from build123d import *

# Parameters (mm, degrees)
SKETCH_1_R      = 1.6
EXTRUDE_1_DEPTH = 3
CHAMFER_1_SIZE  = 4


with BuildPart() as part:
    # 草图1 → 凸台-拉伸1 (new body)
    with BuildSketch(Plane.XY):
        Polygon((-20.3, 16.9), (-35.3, 16.9), (-35.3, 8), (-31.3, 4), (-31.3, -6), (-35.3, -10), (-35.3, -18), (-31.3, -22), (-31.3, -32), (-35.3, -36), (-35.3, -52.9), (-20.3, -52.9), (-14.587407973, -56.9), (-8.874815946, -52.9), (11.874815946, -52.9), (17.587407973, -56.9), (23.3, -52.9), (23.3, -21), (20.3, -18), (23.3, -15), (23.3, 16.9), (17.587407973, 20.9), (11.874815946, 16.9), (-8.874815946, 16.9), (-14.587407973, 20.9), align=None)
        with Locations((-27.8, -47)):
            Circle(SKETCH_1_R, mode=Mode.SUBTRACT)
        with Locations((-27.8, -39)):
            Circle(SKETCH_1_R, mode=Mode.SUBTRACT)
        with BuildLine():
            ThreePointArc((-20.8, -30), (-23.3, -32.5), (-25.8, -30))
            Line((-25.8, -30), (-25.8, -24))
            ThreePointArc((-25.8, -24), (-23.3, -21.5), (-20.8, -24))
            Line((-20.8, -24), (-20.8, -30))
        make_face(mode=Mode.SUBTRACT)
        with BuildLine():
            Line((13.2, -46.9), (-13.2, -46.9))
            ThreePointArc((-13.2, -46.9), (-14.25, -47.95), (-15.3, -46.9))
            Line((-15.3, -46.9), (-15.3, -25.1))
            ThreePointArc((-15.3, -25.1), (-14.25, -24.05), (-13.2, -25.1))
            Line((-13.2, -25.1), (13.2, -25.1))
            ThreePointArc((13.2, -25.1), (14.25, -24.05), (15.3, -25.1))
            Line((15.3, -25.1), (15.3, -46.9))
            ThreePointArc((15.3, -46.9), (14.25, -47.95), (13.2, -46.9))
        make_face(mode=Mode.SUBTRACT)
        with Locations((-27.8, -14)):
            Circle(SKETCH_1_R, mode=Mode.SUBTRACT)
        with BuildLine():
            Line((-25.8, -4), (-25.8, 2))
            ThreePointArc((-25.8, 2), (-23.3, 4.5), (-20.8, 2))
            Line((-20.8, 2), (-20.8, -4))
            ThreePointArc((-20.8, -4), (-23.3, -6.5), (-25.8, -4))
        make_face(mode=Mode.SUBTRACT)
        with Locations((-27.8, 11)):
            Circle(SKETCH_1_R, mode=Mode.SUBTRACT)
        with BuildLine():
            Line((13.2, -10.9), (-13.2, -10.9))
            ThreePointArc((-13.2, -10.9), (-14.25, -11.95), (-15.3, -10.9))
            Line((-15.3, -10.9), (-15.3, 10.9))
            ThreePointArc((-15.3, 10.9), (-14.25, 11.95), (-13.2, 10.9))
            Line((-13.2, 10.9), (13.2, 10.9))
            ThreePointArc((13.2, 10.9), (14.25, 11.95), (15.3, 10.9))
            Line((15.3, 10.9), (15.3, -10.9))
            ThreePointArc((15.3, -10.9), (14.25, -11.95), (13.2, -10.9))
        make_face(mode=Mode.SUBTRACT)
    extrude(amount=EXTRUDE_1_DEPTH)

    # 倒角1
    chamfer_1_edges = [part.edges().sort_by_distance(p)[0] for p in [
        (-35.3, 16.9, 1.5),
        (-35.3, -52.9, 1.5),
    ]]
    chamfer(chamfer_1_edges, length=CHAMFER_1_SIZE)


solid = part.part
Build history of the part. All positions in model axes, mm. A direction names the side the tool comes from. Round coordinates to 2 decimals unless told otherwise and drop trailing zeros. Write each loop counter-clockwise with the first axis right and the second up, starting at its lowest first coordinate (ties: lowest second). Pieces come first, ordered by that corner, then holes. Notation, with made-up numbers: (79.5, 46.25) -> (120.5, 46.25) arc R15 cw to (120.5, 70.25) -> close; hole circle Ø3 at (55, 69). An arc over 180 degrees is marked (long way). Use one line per item in the form item = value.
Q1. Band-saw the part on B-B, the plane y = -39. Write the cut outline in (x, z).
Conclusion:
outline = (-35.3, 0) -> (-29.4, 0) -> (-29.4, 3) -> (-35.3, 3) -> close; (-26.2, 0) -> (-15.3, 0) -> (-15.3, 3) -> (-26.2, 3) -> close; (15.3, 0) -> (23.3, 0) -> (23.3, 3) -> (15.3, 3) -> close
Q2. Band-saw the part on D-D, the plane x = -27.8. Write the cut outline in (y, z).
Conclusion:
outline = (-52.9, 0) -> (-48.6, 0) -> (-48.6, 3) -> (-52.9, 3) -> close; (-45.4, 0) -> (-40.6, 0) -> (-40.6, 3) -> (-45.4, 3) -> close; (-37.4, 0) -> (-15.6, 0) -> (-15.6, 3) -> (-37.4, 3) -> close; (-12.4, 0) -> (9.4, 0) -> (9.4, 3) -> (-12.4, 3) -> close; (12.6, 0) -> (16.9, 0) -> (16.9, 3) -> (12.6, 3) -> close
Q3. Drill centre lines: L1, parallel to X at y = -0.5, z = 1.6; L2, parallel to Y at x = 0, z = 1.35; L3, parallel to Y at x = -27.8, z = 0.85. Where is each one in solid material? Low to high.
Conclusion:
L1 = -31.3 to -25.8, -20.8 to -15.3, 15.3 to 23.3
L2 = -52.9 to -46.9, -25.1 to -10.9, 10.9 to 16.9
L3 = -52.9 to -48.6, -45.4 to -40.6, -37.4 to -15.6, -12.4 to 9.4, 12.6 to 16.9
Q4. Band-saw the part on A-A, the plane x = -6.5. Write the cut outline in (y, z).
Conclusion:
outline = (-52.9, 0) -> (-46.9, 0) -> (-46.9, 3) -> (-52.9, 3) -> close; (-25.1, 0) -> (-10.9, 0) -> (-10.9, 3) -> (-25.1, 3) -> close; (10.9, 0) -> (16.9, 0) -> (16.9, 3) -> (10.9, 3) -> close
Q5. Two-plate mould, pull along X, no slides. Class faces 1 (the flat face through (-33.3, -34, 1.5)), 2 (the flat face through (-26, 16.9, 1)), 3 (the flat face through (0, -25.1, 1)): released by +X, released by -X, zero draft, split by the parting line, or undercut.
Conclusion:
face_1 = released by -X
face_2 = zero draft
face_3 = undercut
Q6. Drop flat-ended pins along their axis: P1, Ø0.9, axis at x = 6, z = 1, coming from the +Y side; P2, Ø1.5, axis at y = -27, z = 1.5, coming from the -X side; P3, Ø1, axis at x = -5, z = 2, coming from the -Y side. Give the stop position or say it passes through.
Conclusion:
P1 = 16.9
P2 = -31.3
P3 = -52.9
Q7. Band-saw the part on C-C, the plane y = -14. Write the cut outline in (x, z).
Conclusion:
outline = (-35.3, 0) -> (-29.4, 0) -> (-29.4, 3) -> (-35.3, 3) -> close; (-26.2, 0) -> (23.3, 0) -> (23.3, 3) -> (-26.2, 3) -> close
Q8. Tool access for faces 4 (the flat face through (-25.8, -1, 1)), 5 (the flat face through (-33.3, -8, 1.5)), 6 (the flat face through (-11.69, 18.87, 1.48)), 7 (the flat face through (21.8, -19.5, 1.5)), 8 (the flat face through (23.3, -37, 1)): list every direction of +Z, -Z, +X, -X, +Y, -Y with a clear straight run to the whole face (end or side of a thin tool).
Conclusion:
face_4 = +Z, -Z
face_5 = +Z, -Z, -X
face_6 = +Z, -Z, +Y
face_7 = +Z, -Z, +X
face_8 = +Z, -Z, +X, +Y, -Y
